Read the model definition and answer for the solid it produces. Units are mm, in the model's axes. A direction names the side the tool comes from. Give positions to 0.01 mm unless a question says otherwise; leave off trailing zeros. Order: outer loops, then holes, each group sorted by start corner. A loop starts at its lowest first (then second) coordinate and runs counter-clockwise, first axis right, second up. Notation, with made-up numbers: (17.25, 25.5) -> (74.25, 25.5) arc R20 ccw to (74.25, 35.5) -> close; hole circle Ø6 at (-13.75, 27.25). An arc over 180 degrees is marked (long way). Use one line per item in the form item = value.
```python
from build123d import *

# Parameters (mm, degrees)
EXTRUDE_1_DEPTH      = 20
SKETCH_2_W           = 18.9
SKETCH_2_H           = 20
EXTRUDE_2_DEPTH      = 4
SKETCH_3_W           = 15
SKETCH_3_H           = 4
EXTRUDE_3_DEPTH      = 39
SKETCH_4_W           = 19
SKETCH_4_H           = 4
EXTRUDE_4_DEPTH      = 16
SKETCH_5_W           = 4
SKETCH_5_H           = 15
EXTRUDE_5_DEPTH      = 20
EXTRUDE_5_DEPTH_BACK = 15
SKETCH_6_W           = 19
SKETCH_6_H           = 4
EXTRUDE_6_DEPTH      = 16
SKETCH_7_R           = 1.8
CUT_EXTRUDE_1_DEPTH  = 16
SKETCH_8_R           = 1.8
CUT_EXTRUDE_2_DEPTH  = 16
SKETCH_9_R           = 1.8
CUT_EXTRUDE_3_DEPTH  = 16


with BuildPart() as part:
    # Sketch 1 → Extrude 1 (new body)
    with BuildSketch(Plane(origin=(0, 0, 0), x_dir=(1, 0, 0), z_dir=(0, 1, 0))):
        Polygon((8.973333333, -3.090335191), (8.973333333, 0.909664809), (-6.026666667, 0.909664809), (-6.026666667, 15.909664809), (8.973333333, 15.909664809), (8.973333333, 19.909664809), (-4.573333333, 19.909664809), (-10.026666667, 19.909664809), (-10.026666667, 0.495974831), (-10.026666667, -3.090335191), align=None)
    extrude(amount=EXTRUDE_1_DEPTH)



with BuildPart() as body_2:
    # Sketch 2 → Extrude 2 (new body)
    with BuildSketch(Plane(origin=(8.973333333, 0, 0), x_dir=(0, 0, -1), z_dir=(1, 0, 0))):
        with Locations((6.359664809, 10)):
            Rectangle(SKETCH_2_W, SKETCH_2_H)
    extrude(amount=EXTRUDE_2_DEPTH)


with BuildPart() as part_1:
    add(part.part)

    add(body_2.part)  # Extrude 3 merges body 2
    # Sketch 3 → Extrude 3 (add)
    with BuildSketch(Plane.ZY.offset(10.026666667)):
        with Locations((-8.409664809, 37)):
            Rectangle(SKETCH_3_W, SKETCH_3_H)
        Polygon((-0.909664809, 20), (3.090335191, 20), (3.090335191, 39), (-0.909664809, 39), (-0.909664809, 35), align=None)
    extrude(amount=-EXTRUDE_3_DEPTH)

    # Sketch 4 → Extrude 4 (add)
    with BuildSketch(Plane(origin=(12.973333333, 0, 0), x_dir=(0, 0, -1), z_dir=(1, 0, 0))):
        with Locations((6.409664809, 18)):
            Rectangle(SKETCH_4_W, SKETCH_4_H)
    extrude(amount=EXTRUDE_4_DEPTH)

    # Sketch 5 → Extrude 5 (add, two sides)
    with BuildSketch(Plane(origin=(0, 0, -15.909664809), x_dir=(-1, 0, 0), z_dir=(0, 0, -1))) as extrude_5_sk:
        Polygon((6.026666667, 35), (10.026666667, 35), (10.026666667, 39), (-8.973333333, 39), (-8.973333333, 35), align=None)
        with Locations((8.026666667, 27.5)):
            Rectangle(SKETCH_5_W, SKETCH_5_H)
    extrude(amount=EXTRUDE_5_DEPTH)
    extrude(extrude_5_sk.sketch, amount=-EXTRUDE_5_DEPTH_BACK)

    # Sketch 6 → Extrude 6 (add)
    with BuildSketch(Plane(origin=(0, 0, -19.909664809), x_dir=(-1, 0, 0), z_dir=(0, 0, -1))):
        with Locations((0.526666667, 18)):
            Rectangle(SKETCH_6_W, SKETCH_6_H)
    extrude(amount=EXTRUDE_6_DEPTH)

    # Sketch 7 → Cut-Extrude 1 (cut)
    with BuildSketch(Plane.XY.offset(3.090335191)):
        with Locations((21.473333333, 27.5)):
            Circle(SKETCH_7_R)
    extrude(amount=-CUT_EXTRUDE_1_DEPTH, mode=Mode.SUBTRACT)

    # Sketch 8 → Cut-Extrude 2 (cut)
    with BuildSketch(Plane.ZY.offset(10.026666667)):
        with Locations((-28.409664809, 27.5)):
            Circle(SKETCH_8_R)
        with Locations((-8.409664809, 7.5)):
            Circle(SKETCH_8_R)
    extrude(amount=-CUT_EXTRUDE_2_DEPTH, mode=Mode.SUBTRACT)

    # Sketch 9 → Cut-Extrude 3 (cut)
    with BuildSketch(Plane.XY.offset(3.090335191)):
        with Locations((1.473333333, 7.5)):
            Circle(SKETCH_9_R)
    extrude(amount=-CUT_EXTRUDE_3_DEPTH, mode=Mode.SUBTRACT)


solid = part_1.part
```
Item 1: Determine the mould class of faces 1 (the flat face through (5, 39, -12)), 2 (the cylindrical face through (22.44, 29.02, 1.12)), 3 (the flat face through (-10.027, 24, -12)) for opening direction Y: +Y half, -Y half, draft (parallel to the pull), parting line (faces both ways), or undercut.
Checks:
face_1 = +Y half
face_2 = undercut
face_3 = draft
Item 2: The part is cut by section C-C on z = -22. Give the vertices of the cut face in (x, y).
Checks:
outline = (-10.03, 16) -> (8.97, 16) -> (8.97, 20) -> (-6.03, 20) -> (-6.03, 35) -> (8.97, 35) -> (8.97, 39) -> (-10.03, 39) -> close
Item 3: Straight lines are drawn through the part: L1, parallel to X at y = 4, z = -15; L2, parallel to Y at x = 4.5, z = -17.5; L3, parallel to Z at x = 5.5, y = 13.5. For each, find the intervals that lie inside material, in ascending order. Write a range as from..to.
Checks:
L1 = -10.03..-6.03, 8.97..12.97
L2 = 0..20, 35..39
L3 = -19.91..-15.91, -0.91..3.09
Item 4: The part is cut by section A-A on y = 7.5. Give the vertices of the cut face in (x, z), and give its area (3 significant figures).
Checks:
outline = (-10.03, -19.91) -> (8.97, -19.91) -> (8.97, -15.91) -> (-6.03, -15.91) -> (-6.03, -10.21) -> (-10.03, -10.21) -> close; (-10.03, -6.61) -> (-6.03, -6.61) -> (-6.03, -0.91) -> (-0.33, -0.91) -> (-0.33, 3.09) -> (-10.03, 3.09) -> close; (3.27, -0.91) -> (8.97, -0.91) -> (8.97, -15.81) -> (12.97, -15.81) -> (12.97, 3.09) -> (3.27, 3.09) -> close
area = 259 mm²
Item 5: Given pin 1 Ø2 at (x, y) = (19.5, 18) entering from -Z; pin 2 Ø3 at (x, y) = (1.47, 7.5) entering from +Z; pin 3 Ø4 at (x, y) = (18, 12.5) entering from +Z; pin 4 Ø3 at (x, z) = (2.5, -14) entering from -Y, each flat-ended and moving along its own axis, determine where each tip first touches the part or whether it passes through.
Checks:
pin_1 = -15.91
pin_2 = -15.91
pin_3 = through
pin_4 = 35
Item 6: The part is cut by section D-D on x = 25. Give the vertices of the cut face in (y, z).
Checks:
outline = (16, -15.91) -> (20, -15.91) -> (20, -0.91) -> (35, -0.91) -> (35, -15.91) -> (39, -15.91) -> (39, 3.09) -> (16, 3.09) -> close
Item 7: The part is cut by section B-B on x = 4.5. Give the vertices of the cut face in (y, z).
Checks:
outline = (0, -19.91) -> (16, -19.91) -> (16, -35.91) -> (20, -35.91) -> (20, -15.91) -> (0, -15.91) -> close; (0, -0.91) -> (35, -0.91) -> (35, -35.91) -> (39, -35.91) -> (39, 3.09) -> (0, 3.09) -> close
Item 8: Which of the six approach directions +Z, -Z, +X, -X, +Y, -Y give full straight-line access (tool end or side, diameter ignored) to faces 4 (the cylindrical face through (-8.055, 5.743, -8.8)), 5 (the flat face through (1, 10, -15.91)), 6 (the flat face through (8.973, 37, -26)), 7 (the flat face through (0, 8, -19.91))?
Checks:
face_4 = -X
face_5 = -Y
face_6 = -Z, +X, +Y, -Y
face_7 = -Z, +X, -X, -Y
